Geometry: final body of the model. Coordinates: model frame, mm. A direction names the side the tool comes from. Give positions to 0.01 mm unless a question says otherwise; leave off trailing zeros. Loops run counter-clockwise (first coordinate to the right, second up) from the corner with the lowest first, then second, coordinate; pieces in that order, holes last.
from build123d import *

# Parameters (mm, degrees)
SKETCH1_W           = 56.4
SKETCH1_H           = 56.4
BOSS_EXTRUDE1_DEPTH = 40
SKETCH2_R           = 2.75
CUT_EXTRUDE1_DEPTH  = 79.317122537
CUT_EXTRUDE3_DEPTH  = 79.317122537
SKETCH5_W           = 14.63
SKETCH5_H           = 8.2
CUT_EXTRUDE4_DEPTH  = 30
FILLET1_R           = 2
FILLET2_R           = 2
FILLET3_R           = 1


with BuildPart() as part:
    # Sketch1 → Boss-Extrude1 (new body)
    with BuildSketch(Plane(origin=(0, 0, 0), x_dir=(0, 0, -1), z_dir=(1, 0, 0))):
        with Locations((10.777070064, -26.703184713)):
            Rectangle(SKETCH1_W, SKETCH1_H)
    extrude(amount=BOSS_EXTRUDE1_DEPTH)

    # Sketch2 → Cut-Extrude1 (cut, through all)
    with BuildSketch(Plane(origin=(40, 0, 0), x_dir=(0, 0, -1), z_dir=(1, 0, 0))):
        with Locations((-12.792929936, -3.133184713)):
            Circle(SKETCH2_R)
        with Locations(Location((-12.792929936, -50.273184713, 0), (0, 0, 180))):
            Circle(SKETCH2_R)
        with Locations(Location((34.347070064, -3.133184713, 0), (0, 0, 180))):
            Circle(SKETCH2_R)
        with Locations((34.347070064, -50.273184713)):
            Circle(SKETCH2_R)
    extrude(amount=-CUT_EXTRUDE1_DEPTH, mode=Mode.SUBTRACT)

    # Sketch4 → Cut-Extrude3 (cut, through all)
    with BuildSketch(Plane(origin=(40, 0, 0), x_dir=(0, 0, -1), z_dir=(1, 0, 0))):
        with BuildLine():
            Line((10.777070064, -6.703184713), (-17.422929936, -6.703184713))
            Line((-17.422929936, -6.703184713), (-17.422929936, -46.703184713))
            Line((-17.422929936, -46.703184713), (10.777070064, -46.703184713))
            ThreePointArc((10.777070064, -46.703184713), (30.777070064, -26.703184713), (10.777070064, -6.703184713))
        make_face()
    extrude(amount=-CUT_EXTRUDE3_DEPTH, mode=Mode.SUBTRACT)

    # Sketch5 → Cut-Extrude4 (cut)
    with BuildSketch(Plane(origin=(40, 0, 0), x_dir=(0, 0, -1), z_dir=(1, 0, 0))):
        with Locations((-10.107929936, -2.603184713)):
            Rectangle(SKETCH5_W, SKETCH5_H)
        with Locations((-10.107929936, -50.803184713)):
            Rectangle(SKETCH5_W, SKETCH5_H)
    extrude(amount=-CUT_EXTRUDE4_DEPTH, mode=Mode.SUBTRACT)

    # Fillet1
    fillet1_edges = [part.edges().sort_by_distance(p)[0] for p in [
        (10, -2.603184713, 2.792929936),
        (10, -50.803184713, 2.792929936),
    ]]
    fillet(fillet1_edges, radius=FILLET1_R)

    # Fillet2
    fillet2_edges = [part.edges().sort_by_distance(p)[0] for p in [
        (40, -2.603184713, 2.792929936),
        (40, -50.803184713, 2.792929936),
    ]]
    fillet(fillet2_edges, radius=FILLET2_R)

    # Fillet3
    fillet3_edges = [part.edges().sort_by_distance(p)[0] for p in [
        (10, -2.603184713, 17.422929936),
        (10, -50.803184713, 17.422929936),
    ]]
    fillet(fillet3_edges, radius=FILLET3_R)


solid = part.part
Item 1: Section query B-B on x = 11. Return loops of the section in (y, z), plus the area to 3 significant figures.
Values follow:
outline: (-54.9, -38.98) - (1.5, -38.98) - (1.5, 3.06) - (-6.7, 3.06) - (-6.7, -10.78) arc R20 cw to (-46.7, -10.78) - (-46.7, 3.06) - (-54.9, 3.06) - close; hole circle Ø5.5 at (-50.27, -34.35); hole circle Ø5.5 at (-3.13, -34.35)
area: 1,140 mm2
Item 2: Section query D-D on x = 3.5. Return loops of the section in (y, z).
Values follow:
outline: (-54.9, -38.98) - (1.5, -38.98) - (1.5, 17.42) - (-6.7, 17.42) - (-6.7, -10.78) arc R20 cw to (-46.7, -10.78) - (-46.7, 17.42) - (-54.9, 17.42) - close; hole circle Ø5.5 at (-50.27, -34.35); hole circle Ø5.5 at (-50.27, 12.79); hole circle Ø5.5 at (-3.13, -34.35); hole circle Ø5.5 at (-3.13, 12.79)
Item 3: Section query C-C on z = -32.5. Return loops of the section in (x, y), plus the area to 3 significant figures.
Values follow:
outline: (0, -54.9) - (40, -54.9) - (40, -52.31) - (0, -52.31) - close; (0, -48.24) - (40, -48.24) - (40, -5.17) - (0, -5.17) - close; (0, -1.1) - (40, -1.1) - (40, 1.5) - (0, 1.5) - close
area: 1,930 mm2
Item 4: Set-up query: faces 5 (the face through (25, -51, 2.793)), 6 (the face through (16, -6.703, -3)), 7 (the face through (0, -29, -32)). Return all of +Z, -Z, +X, -X, +Y, -Y with unobstructed straight access to the full face (end or side cutting, diameter ignored); none if empty.
Values follow:
face 5: +Z, +X, +Y, -Y
face 6: +Z, +X, -X
face 7: +Z, -Z, -X, +Y, -Y
Item 5: Ray query, probe 1 along Y at (x, z) = (38, -32); probe 2 along Y at (x, z) = (7, 10.5); probe 3 along Z at (x, y) = (7, -2). Return the intervals inside material, ascending.
Values follow:
probe 1: y = -54.9 to -51.71, -48.84 to -4.57, -1.7 to 1.5
probe 2: y = -54.9 to -51.79, -48.75 to -46.7, -6.7 to -4.65, -1.61 to 1.5
probe 3: z = -38.98 to -36.85, -31.84 to 10.29, 15.3 to 17.42
Item 6: Section query A-A on z = -1. Return loops of the section in (x, y), plus the area to 3 significant figures.
Values follow:
outline: (0, -54.9) - (40, -54.9) - (40, -46.7) - (0, -46.7) - close; (0, -6.7) - (40, -6.7) - (40, 1.5) - (0, 1.5) - close
area: 656 mm2
Item 7: Draft query along Z for faces 1 (the face through (40, -26, -32)), 2 (the face through (20, -27, -38.977)), 3 (the face through (20.28, -47.547, -33.989)), 4 (the face through (39.4, -50.75, 2.22)). Return one class per face: +Z half, -Z half, draft (parallel to the pull), parting line (faces both ways), or undercut.
Values follow:
face 1: draft
face 2: -Z half
face 3: undercut
face 4: +Z half
Item 8: Pin query (flat end, axial travel): pin 1 (2.5 mm diameter, centred on y = -50, z = 11, fed in from +X); pin 2 (2 mm diameter, centred on x = 28, y = -39.5, fed in from +Z); pin 3 (9 mm diameter, centred on x = 20.5, y = -4.5, fed in from +Z); pin 4 (5 mm diameter, centred on y = -3.13, z = 12.79, fed in from +X). Return the tip coordinate at first contact, or that it passes through.
Values follow:
pin 1: stops at x = 10
pin 2: stops at z = -25.26
pin 3: stops at z = 2.79
pin 4: passes through
